For this review, take the finished solid that the model builds, in its own axes (mm). Face numbers are marked on the shaded views. A direction names the side the tool comes from. Coordinates: 2 decimals unless noted, no trailing zeros. Write each loop counter-clockwise with the first axis right and the second up, starting at its lowest first coordinate (ties: lowest second). Pieces come first, ordered by that corner, then holes. Notation, with made-up numbers: (80.5, 44) - (132.5, 44) arc R19 cw to (132.5, 55) - close; hole circle Ø8 at (20.5, -11.5). An arc over 180 degrees is marked (long way). Use one line per item in the form item = value. Start each with the question number.
1) Insertion check: P1, Ø3, axis at x = 35, z = 15, coming from the -Y side; P2, Ø7.5, axis at x = 32.5, z = 13, coming from the -Y side; P3, Ø7, axis at x = 0, z = -64.03, coming from the -Y side; P4, Ø0.6, axis at x = 11, y = 1.5, coming from the -Z side. Each pin has a flat end and moves straight along its axis. Give the tip position at first contact, or say it passes through.
2) We need section B-B (z = 0). Count the separate pieces of the cut face and the enclosed holes in it, plus the area to 3 significant figures.
3) We need section D-D (x = -79). Give the boundary of the cut face in (y, z), plus the area to 3 significant figures.
4) Mouldability with a two-part tool opening along Y and no side actions: class the marked faces 1 and 2 as pulls with the +Y half, pulls with the -Y half, needs draft (parallel to the pull), parting line crosses it, or undercut.
5) For L1, parallel to X at y = 1.5, z = 0; L2, parallel to X at y = 0.8, z = 15; L3, parallel to Z at x = 27.5, y = -0.75, list the stretches that pass through material, from the lowest coordinate up. Write a range as from..to.
6) We need section C-C (z = 79). Give the boundary of the cut face in (x, y), plus the area to 3 significant figures.
7) Tool access review of the marked faces 3 and 4: name each direction out of +Z, -Z, +X, -X, +Y, -Y from which nothing blocks a thin tool from reaching the whole face with its end or side.
8) We need section A-A (x = 0). Give the boundary of the cut face in (y, z), plus the area to 3 significant figures.
```python
from build123d import *
from build123d.topology import SkipClean

# Parameters (mm, degrees)
SKETCH_1_R            = 85.5
SKETCH_1_R_2          = 2.65
EXTRUDE_1_DEPTH       = 2
SKETCH_2_W            = 40
SKETCH_2_H            = 100
CUT_EXTRUDE_2_DEPTH   = 2
SKETCH_4_R            = 2.65
CUT_EXTRUDE_3_DEPTH   = 2
SKETCH_5_W            = 15
SKETCH_5_H            = 100
EXTRUDE_2_DEPTH       = 2
SKETCH_7_R            = 2.65
CUT_EXTRUDE_4_DEPTH   = 2
EXTRUDE_4_OUTLINE_R   = 72.5
EXTRUDE_4_OUTLINE_R_2 = 2.65
EXTRUDE_4_OUTLINE_W   = 100
EXTRUDE_4_OUTLINE_H   = 100
EXTRUDE_4_DEPTH       = 2


# Read off the part's stored shape, not the designer's step: 凸台-拉伸4
with BuildPart() as part:
    # 草图1 → 凸台-拉伸1 (new body)
    with BuildSketch(Plane(origin=(0, 0, 0), x_dir=(1, 0, 0), z_dir=(0, 1, 0))):
        with Locations(Location((0, 0, 0), (0, 0, 270))):
            Circle(SKETCH_1_R)
        with Locations(Location((0, 79, 0), (0, 0, 270))):
            Circle(SKETCH_1_R_2, mode=Mode.SUBTRACT)
        with Locations(Location((79, 0, 0), (0, 0, 270))):
            Circle(SKETCH_1_R_2, mode=Mode.SUBTRACT)
        with Locations(Location((0, -79, 0), (0, 0, 270))):
            Circle(SKETCH_1_R_2, mode=Mode.SUBTRACT)
        with Locations(Location((-79, 0, 0), (0, 0, 270))):
            Circle(SKETCH_1_R_2, mode=Mode.SUBTRACT)
    extrude(amount=EXTRUDE_1_DEPTH)

    # 草图2 → 切除-拉伸2 (cut)
    with BuildSketch(Plane(origin=(0, 2, 0), x_dir=(1, 0, 0), z_dir=(0, 1, 0))):
        with Locations((-20, 0)):
            Rectangle(SKETCH_2_W, SKETCH_2_H)
        with Locations((20, 0)):
            Rectangle(SKETCH_2_W, SKETCH_2_H)
    extrude(amount=-CUT_EXTRUDE_2_DEPTH, mode=Mode.SUBTRACT)

    # 草图4 → 切除-拉伸3 (cut)
    with BuildSketch(Plane(origin=(0, 2, 0), x_dir=(1, 0, 0), z_dir=(0, 1, 0))):
        with Locations(Location((0, 64.031242374, 0), (0, 0, 270))):
            Circle(SKETCH_4_R)
        with Locations(Location((64.031242374, 0, 0), (0, 0, 270))):
            Circle(SKETCH_4_R)
        with Locations(Location((0, -64.031242374, 0), (0, 0, 270))):
            Circle(SKETCH_4_R)
        with Locations(Location((-64.031242374, 0, 0), (0, 0, 270))):
            Circle(SKETCH_4_R)
    extrude(amount=-CUT_EXTRUDE_3_DEPTH, mode=Mode.SUBTRACT)

    # 草图5 → 凸台-拉伸2 (add)
    with BuildSketch(Plane(origin=(0, 2, 0), x_dir=(1, 0, 0), z_dir=(0, 1, 0))):
        with Locations((-32.5, 0)):
            Rectangle(SKETCH_5_W, SKETCH_5_H)
        with Locations((32.5, 0)):
            Rectangle(SKETCH_5_W, SKETCH_5_H)
    extrude(amount=-EXTRUDE_2_DEPTH)

    # 草图7 → 切除-拉伸4 (cut)
    with BuildSketch(Plane(origin=(0, 2, 0), x_dir=(1, 0, 0), z_dir=(0, 1, 0))):
        with Locations(Location((35, 15, 0), (0, 0, 270))):
            Circle(SKETCH_7_R)
        with Locations(Location((35, -15, 0), (0, 0, 270))):
            Circle(SKETCH_7_R)
        with Locations(Location((-35, -15, 0), (0, 0, 270))):
            Circle(SKETCH_7_R)
        with Locations(Location((-35, 15, 0), (0, 0, 270))):
            Circle(SKETCH_7_R)
    extrude(amount=-CUT_EXTRUDE_4_DEPTH, mode=Mode.SUBTRACT)

    # 凸台-拉伸4 outline → 凸台-拉伸4 (add)
    with SkipClean():  # the faces are left unmerged after this step: merging them gives an invalid solid
        with BuildSketch(Plane.XZ):
            Circle(EXTRUDE_4_OUTLINE_R)
            with Locations((0, -64.031242374)):
                Circle(EXTRUDE_4_OUTLINE_R_2, mode=Mode.SUBTRACT)
            with Locations((-64.031242374, 0)):
                Circle(EXTRUDE_4_OUTLINE_R_2, mode=Mode.SUBTRACT)
            Rectangle(EXTRUDE_4_OUTLINE_W, EXTRUDE_4_OUTLINE_H, mode=Mode.SUBTRACT)
            with Locations((64.031242374, 0)):
                Circle(EXTRUDE_4_OUTLINE_R_2, mode=Mode.SUBTRACT)
            with Locations((0, 64.031242374)):
                Circle(EXTRUDE_4_OUTLINE_R_2, mode=Mode.SUBTRACT)
        extrude(amount=EXTRUDE_4_DEPTH)
    add(part.part.scale(1), mode=Mode.REPLACE)  # the faces are merged on a copy


solid = part.part
```
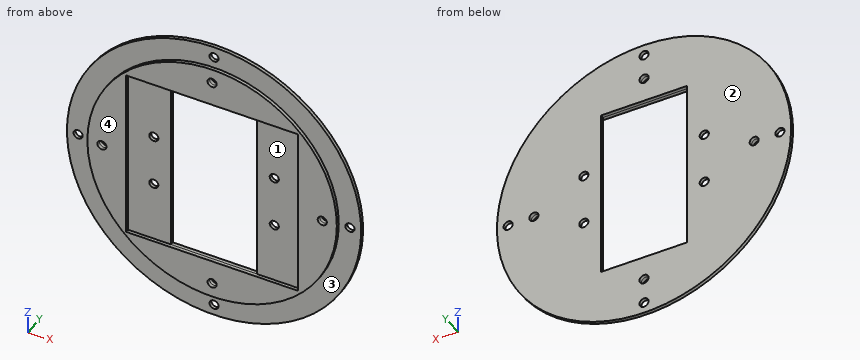
Determined:
q1.P1 = through
q1.P2 = 0
q1.P3 = -2
q1.P4 = -84.83
q2.separate_pieces = 6
q2.enclosed_holes = 0
q2.area = 268 mm²
q3.outline = (0, -32.7) - (2, -32.7) - (2, -2.65) - (0, -2.65) - close; (0, 2.65) - (2, 2.65) - (2, 32.7) - (0, 32.7) - close
q3.area = 120 mm²
q4.face_1 = pulls with the -Y half
q4.face_2 = pulls with the +Y half
q5.L1 = -85.5..-81.65, -76.35..-66.68, -61.38..-25, 25..61.38, 66.68..76.35, 81.65..85.5
q5.L2 = -84.17..-37.65, -32.35..-25, 25..32.35, 37.65..84.17
q5.L3 = -67.08..-50, 50..67.08
q6.outline = (-32.7, 0) - (-2.65, 0) - (-2.65, 2) - (-32.7, 2) - close; (2.65, 0) - (32.7, 0) - (32.7, 2) - (2.65, 2) - close
q6.area = 120 mm²
q7.face_3 = -Y
q7.face_4 = +Z, -Z, +X, -X, -Y
q8.outline = (-2, -72.5) - (0, -72.5) - (0, -76.35) - (2, -76.35) - (2, -66.68) - (-2, -66.68) - close; (-2, -61.38) - (2, -61.38) - (2, -50) - (-2, -50) - close; (-2, 50) - (2, 50) - (2, 61.38) - (-2, 61.38) - close; (-2, 66.68) - (2, 66.68) - (2, 76.35) - (0, 76.35) - (0, 72.5) - (-2, 72.5) - close; (0, -85.5) - (2, -85.5) - (2, -81.65) - (0, -81.65) - close; (0, 81.65) - (2, 81.65) - (2, 85.5) - (0, 85.5) - close
q8.area = 168 mm²
